Geometry: final body of the model. Coordinates: model frame, mm. Round coordinates to 2 decimals unless told otherwise and drop trailing zeros. Write each loop counter-clockwise with the first axis right and the second up, starting at its lowest first coordinate (ties: lowest second). Pieces come first, ordered by that corner, then holes. Notation, with made-up numbers: M 73,41.25 L 104,41.25 A28 cw 104,77.25 Z; hole C 13.5,73.5 d10. An arc over 180 degrees is marked long. Use one line per item in the form item = value. Start each with the question number.
Item 1: Section query A-A (x = -9.38). Return loops of the section in (y, z).
Item 2: Ray query, probe 1 along X at (y, z) = (1, 2.75); probe 2 along Z at (x, y) = (-2, 6). Return the intervals inside material, ascending.
Item 3: Section query D-D (y = 6.5). Return loops of the section in (x, z).
Item 4: Pin query (flat end, axial travel): pin 1 Ø2.5 at (x, y) = (-14.08, 0) entering from +Z; pin 2 Ø2.5 at (x, y) = (0, 16.615) entering from -Z; pin 3 Ø4.5 at (x, y) = (1, -0.5) entering from -Z; pin 4 Ø2 at (x, z) = (6, 1) entering from -Y. Return the tip coordinate at first contact, or that it passes through.
Item 5: Section query B-B (z = 4). State how many separate pieces and enclosed holes the cut face has, and give its area (3 significant figures).
Item 6: Pull-direction query (Y, two-part tool) for faces 1 (the cylindrical face through (1.2, -2.4, 6.7)), 2 (the flat face through (13.24, -4.35, 3.64)), 3 (the flat face through (13.39, 4.33, 3.64)); classes: pulls with the +Y half, pulls with the -Y half, needs draft (parallel to the pull), parting line crosses it, or undercut.
Item 7: Section query C-C (y = -16). Return loops of the section in (x, z).
from build123d import *

# Parameters (mm, degrees)
SKETCH1_R                 = 5.98
BOSS_EXTRUDE1_DEPTH       = 1.15
BOSS_EXTRUDE2_DEPTH       = 5.05
F_3_0MM_DOWEL_HOLE1_D     = 3.06
F_3_0MM_DOWEL_HOLE1_DEPTH = 15
F_3_0MM_DOWEL_HOLE1_TIP   = 0.919316747
SKETCH6_R                 = 0.25
CUT_EXTRUDE1_DEPTH        = 3.96
SKETCH7_R                 = 2.675
CUT_EXTRUDE2_DEPTH        = 3.96
SKETCH8_R                 = 1.19
CUT_EXTRUDE3_DEPTH        = 8.35
SKETCH9_OUTSIDE_W         = 70.76
SKETCH9_OUTSIDE_H         = 75.83
SKETCH9_OUTSIDE_R         = 19.05
CUT_EXTRUDE4_DEPTH        = 8.35


with BuildPart() as part:
    # Sketch1 → Boss-Extrude1 (new body, symmetric)
    with BuildSketch(Plane.XY):
        Circle(SKETCH1_R)
    extrude(amount=BOSS_EXTRUDE1_DEPTH, both=True)

    # Sketch2 → Boss-Extrude2 (add)
    with BuildSketch(Plane.XY.offset(1.15)):
        with BuildLine():
            Line((-3, 26.015), (-4.945, 8.011816273))
            ThreePointArc((-4.945, 8.011816273), (-6.609281124, 6.70087173), (-7.933478152, 5.047115555))
            Line((-7.933478152, 5.047115555), (-23.48, 3))
            ThreePointArc((-23.48, 3), (-26.48, 0), (-23.48, -3))
            Line((-23.48, -3), (-7.933478152, -5.047115555))
            ThreePointArc((-7.933478152, -5.047115555), (-6.609281124, -6.70087173), (-4.945, -8.011816273))
            Line((-4.945, -8.011816273), (-3, -26.015))
            ThreePointArc((-3, -26.015), (0, -29.015), (3, -26.015))
            Line((3, -26.015), (4.945, -8.011816273))
            ThreePointArc((4.945, -8.011816273), (6.609281124, -6.70087173), (7.933478152, -5.047115555))
            Line((7.933478152, -5.047115555), (23.48, -3))
            ThreePointArc((23.48, -3), (26.48, 0), (23.48, 3))
            Line((23.48, 3), (7.933478152, 5.047115555))
            ThreePointArc((7.933478152, 5.047115555), (6.609281124, 6.70087173), (4.945, 8.011816273))
            Line((4.945, 8.011816273), (3, 26.015))
            ThreePointArc((3, 26.015), (0, 29.015), (-3, 26.015))
        make_face()
    extrude(amount=BOSS_EXTRUDE2_DEPTH)

    # Ø3.0mm Dowel Hole1
    with Locations(Plane.XY.offset(6.2)):
        with Locations((0, 0)):
            Hole(F_3_0MM_DOWEL_HOLE1_D / 2, depth=F_3_0MM_DOWEL_HOLE1_DEPTH)
            with Locations((0, 0, -(F_3_0MM_DOWEL_HOLE1_DEPTH + F_3_0MM_DOWEL_HOLE1_TIP / 2))):  # 118° drill point
                Cone(0, F_3_0MM_DOWEL_HOLE1_D / 2, F_3_0MM_DOWEL_HOLE1_TIP, mode=Mode.SUBTRACT)

    # Sketch5 → Revolve1 (revolve)
    with BuildSketch(Plane(origin=(0, 0, 0), x_dir=(1, 0, 0), z_dir=(0, 1, 0))):
        Polygon((2.685, -6.2), (2.685, -7.1), (4.915, -7.1), (5.15, -6.2), align=None)
    revolve(axis=Axis((0, 0, -17.732106559), (0, 0, 1)))

    # Sketch6 → Cut-Extrude1 (cut)
    with BuildSketch(Plane(origin=(0, 0, -1.15), x_dir=(-1, 0, 0), z_dir=(0, 0, -1))):
        with Locations((0, 2.675)):
            Circle(SKETCH6_R)
        with Locations((0.914903883, 2.513677761)):
            Circle(SKETCH6_R)
        with Locations((1.719456856, 2.049168885)):
            Circle(SKETCH6_R)
        with Locations((2.316617955, 1.3375)):
            Circle(SKETCH6_R)
        with Locations((2.634360739, 0.464508875)):
            Circle(SKETCH6_R)
        with Locations((2.634360739, -0.464508875)):
            Circle(SKETCH6_R)
        with Locations((2.316617955, -1.3375)):
            Circle(SKETCH6_R)
        with Locations((1.719456856, -2.049168885)):
            Circle(SKETCH6_R)
        with Locations((0.914903883, -2.513677761)):
            Circle(SKETCH6_R)
        with Locations((0, -2.675)):
            Circle(SKETCH6_R)
        with Locations((-0.914903883, -2.513677761)):
            Circle(SKETCH6_R)
        with Locations((-1.719456856, -2.049168885)):
            Circle(SKETCH6_R)
        with Locations((-2.316617955, -1.3375)):
            Circle(SKETCH6_R)
        with Locations((-2.634360739, -0.464508875)):
            Circle(SKETCH6_R)
        with Locations((-2.634360739, 0.464508875)):
            Circle(SKETCH6_R)
        with Locations((-2.316617955, 1.3375)):
            Circle(SKETCH6_R)
        with Locations((-1.719456856, 2.049168885)):
            Circle(SKETCH6_R)
        with Locations((-0.914903883, 2.513677761)):
            Circle(SKETCH6_R)
    extrude(amount=-CUT_EXTRUDE1_DEPTH, mode=Mode.SUBTRACT)

    # Sketch7 → Cut-Extrude2 (cut)
    with BuildSketch(Plane(origin=(0, 0, -1.15), x_dir=(-1, 0, 0), z_dir=(0, 0, -1))):
        Circle(SKETCH7_R)
    extrude(amount=-CUT_EXTRUDE2_DEPTH, mode=Mode.SUBTRACT)

    # Sketch8 → Cut-Extrude3 (cut, through all)
    with BuildSketch(Plane.XY.offset(6.2)):
        with Locations((0, 11.915)):
            Circle(SKETCH8_R)
        with Locations((0, 16.615)):
            Circle(SKETCH8_R)
        with Locations((0, 21.315)):
            Circle(SKETCH8_R)
        with Locations((0, 26.015)):
            Circle(SKETCH8_R)
        with Locations((0, -26.015)):
            Circle(SKETCH8_R)
        with Locations((0, -21.315)):
            Circle(SKETCH8_R)
        with Locations((0, -16.615)):
            Circle(SKETCH8_R)
        with Locations((0, -11.915)):
            Circle(SKETCH8_R)
        with Locations((-23.48, 0)):
            Circle(SKETCH8_R)
        with Locations((-18.78, 0)):
            Circle(SKETCH8_R)
        with Locations((-14.08, 0)):
            Circle(SKETCH8_R)
        with Locations((-9.38, 0)):
            Circle(SKETCH8_R)
        with Locations((9.38, 0)):
            Circle(SKETCH8_R)
        with Locations((14.08, 0)):
            Circle(SKETCH8_R)
        with Locations((18.78, 0)):
            Circle(SKETCH8_R)
        with Locations((23.48, 0)):
            Circle(SKETCH8_R)
    extrude(amount=-CUT_EXTRUDE3_DEPTH, mode=Mode.SUBTRACT)

    # Sketch9 outside → Cut-Extrude4 (cut, through all)
    with BuildSketch(Plane.XY.offset(6.2)):
        Rectangle(SKETCH9_OUTSIDE_W, SKETCH9_OUTSIDE_H)
        Circle(SKETCH9_OUTSIDE_R, mode=Mode.SUBTRACT)
    extrude(amount=-CUT_EXTRUDE4_DEPTH, mode=Mode.SUBTRACT)


solid = part.part
Working result:
q1.outline = M -4.86,1.15 L -1.19,1.15 L -1.19,6.2 L -4.86,6.2 Z; M 1.19,1.15 L 4.86,1.15 L 4.86,6.2 L 1.19,6.2 Z
q2.probe_1 = -18.13 to -14.73, -13.43 to -10.03, -8.73 to -2.48, 2.48 to 8.73, 10.03 to 13.43, 14.73 to 18.13
q2.probe_2 = 1.15 to 6.2
q3.outline = M -6.81,1.15 L 6.81,1.15 L 6.81,6.2 L -6.81,6.2 Z
q4.pin_1 = 6.2
q4.pin_2 = 1.15
q4.pin_3 = -1.15
q4.pin_4 = -7.97
q5.separate_pieces = 1
q5.enclosed_holes = 9
q5.area = 571 mm²
q6.face_1 = undercut
q6.face_2 = pulls with the -Y half
q6.face_3 = pulls with the +Y half
q7.outline = M -4.08,1.15 L -1.02,1.15 L -1.02,6.2 L -4.08,6.2 Z; M 1.02,1.15 L 4.08,1.15 L 4.08,6.2 L 1.02,6.2 Z
